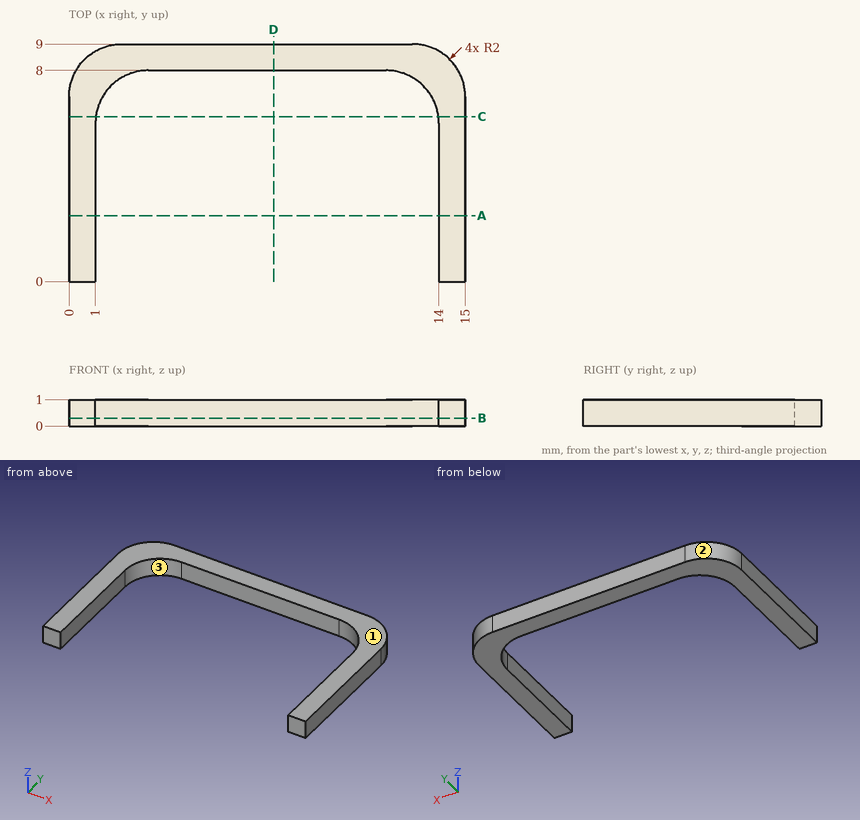
The figure shows three views and two pictorial views of one solid part (mm, origin at its lowest corner). Answer the questions. Give positions to 0.01 mm unless a question says otherwise; leave off trailing zeros. Write each loop counter-clockwise with the first axis right and the second up, starting at its lowest first coordinate (ties: lowest second). Pieces come first, ordered by that corner, then holes. Notation, with made-up numbers: (3, -25) - (25, -25) arc R30 cw to (25, 10) - close; hole circle Ø10 at (3.5, 66.25). An arc over 180 degrees is marked (long way). Return JSON: item names as keys, results as strings.
Q1. A cutting plane is placed at D-D, the plane x = 7.75. Determine the outline of the cut face in (y, z), and give its area (3 significant figures).
Reply:
{"outline": "(8, 0) - (9, 0) - (9, 1) - (8, 1) - close", "area": "1.00 mm²"}
Q2. Consider line 1 along X through (y, z) = (6, 0.25); line 2 along Y through (x, z) = (5.75, 0.8); line 3 along X through (y, z) = (7.75, 0.85). Determine where each line is inside the solid, lowest interval first. Write a range as [from, to].
Reply:
{"line 1": "[0, 1], [14, 15]", "line 2": "[8, 9]", "line 3": "[0.15, 2.03], [12.97, 14.85]"}
Q3. For a pull along X with two mould halves and no side action, classify the marked faces 1, 2 and 3 as released by +X, released by -X, zero draft, split by the parting line, or undercut.
Reply:
{"face 1": "zero draft", "face 2": "released by -X", "face 3": "undercut"}
Q4. A cutting plane is placed at C-C, the plane y = 6.25. Determine the outline of the cut face in (x, z).
Reply:
{"outline": "(0, 0) - (1.02, 0) - (1.02, 1) - (0, 1) - close; (13.98, 0) - (15, 0) - (15, 1) - (13.98, 1) - close"}
Q5. A cutting plane is placed at B-B, the plane z = 0.3. Determine the outline of the cut face in (x, y), and give its area (3 significant figures).
Reply:
{"outline": "(0, 0) - (1, 0) - (1, 6) arc R2 cw to (3, 8) - (12, 8) arc R2 cw to (14, 6) - (14, 0) - (15, 0) - (15, 7) arc R2 ccw to (13, 9) - (2, 9) arc R2 ccw to (0, 7) - close", "area": "31.0 mm²"}
Q6. A cutting plane is placed at A-A, the plane y = 2.5. Determine the outline of the cut face in (x, z).
Reply:
{"outline": "(0, 0) - (1, 0) - (1, 1) - (0, 1) - close; (14, 0) - (15, 0) - (15, 1) - (14, 1) - close"}
